Autodesk Inventor part; units mm, degrees
ref_plane "YZ Plane" through (0, 0, 0) normal (1, 0, 0) x (0, 1, 0)
ref_plane "XZ Plane" through (0, 0, 0) normal (0, 1, 0) x (-1, 0, 0)
ref_plane "XY Plane" through (0, 0, 0) normal (0, 0, 1) x (1, 0, 0)
sketch "スケッチ1" plane through (0, 0, 0) normal (0, 1, 0) x (-1, 0, 0)
  line L0 (0, 0) -> (0, -112.7681) construction
  line L1 (0, -112.7681) -> (0, 117.0869) construction
  line L2 (0, -1.5) -> (5, -1.5) construction
  line L3 (5, -1.5) -> (5, 1.5)
  line L4 (0, 1.5) -> (5, 1.5) construction
  line L5 (7.5, -1.5) -> (7.5, 1.5)
  line L6 (7.5, -1.5) -> (5, 1.5) construction
  line L7 (5, -1.5) -> (7.5, 1.5) construction
  line L8 (7.116, -1.5) -> (5.384, 1.5) construction
  line L9 (5.384, -1.5) -> (7.116, 1.5) construction
  line L10 (6.25, 0) -> (6.25, 1.5) construction
  line L11 (6.75, -0.866) -> (6.75, -1.5)
  line L12 (5.75, -0.866) -> (5.75, -1.5)
  line L13 (6.75, 0.866) -> (6.75, 1.5)
  line L14 (5.75, 0.866) -> (5.75, 1.5)
  line L15 (5, 1.5) -> (5.75, 1.5)
  line L16 (6.75, 1.5) -> (7.5, 1.5)
  arc A0 (6.75, 0.866) -> (5.75, 0.866) centre (6.25, 0) ccw
  arc A1 (5.75, 0.866) -> (5.75, -0.866) centre (6.25, 0) ccw
  arc A2 (5.75, -0.866) -> (6.8902, -0.7682) centre (6.25, 0) ccw
  arc A3 (6.8902, -0.7682) -> (6.75, 0.866) centre (6.25, 0) ccw
  line L17 (5, -1.5) -> (5.75, -1.5)
  line L18 (6.75, -1.5) -> (7.5, -1.5)
  point P0 (6.25, 0)
  dimension "d0" = 5
  dimension "d1" = 1.5
  dimension "d2" = 1.5
  dimension "d3" = 7.5
  dimension "d6" = 30
  dimension "d7" = 30
  dimension "d11" = 1
revolve "回転2" add sketch "スケッチ1" angle 360 about axis through (0, 0, 0) along (0, 0, -1)
properties part number "ベアリング10.15" material "ステンレス鋼"
The model under review builds one solid part; all positions refer to its coordinate system, in mm. Round coordinates to 2 decimals unless told otherwise and drop trailing zeros. Write each loop counter-clockwise with the first axis right and the second up, starting at its lowest first coordinate (ties: lowest second). Pieces come first, ordered by that corner, then holes.
(1) Insertion check: pin 1 (1.5 mm diameter, centred on y = 4, z = 0, fed in from -X). The pin has a flat end and moves straight along its axis. Give the tip position at first contact, or say it passes through.
(2) Mouldability with a two-part tool opening along Y and no side actions: class faces 1 (the cylindrical face through (0.75, 5.7, -1.19)), 2 (the cylindrical face through (7.493, -0.33, 0.021)), 3 (the flat face through (7, 1, 1.5)) as +Y half, -Y half, draft (parallel to the pull), parting line (faces both ways), or undercut.
(3) We need section A-A on x = 0. Give the boundary of the cut face in (y, z), and give its area (3 significant figures).
(4) We need section C-C on z = -0.2. Give the boundary of the cut face in (x, y), and give its area (3 significant figures).
(5) Wall thickness on L1, parallel to Y at x = 0, z = 1.1; L2, parallel to Y at x = 0, z = -0.55; L3, parallel to X at y = 4, z = 0.7: over which ranges is each line inside the solid? List them lowest first.
Findings below:
1. pin 1: stops at x = -6.76
2. face 1: undercut
2. face 2: parting line
2. face 3: draft
3. outline: (-7.5, -1.5) - (-6.75, -1.5) - (-6.75, -0.87) arc R1 ccw to (-5.75, -0.87) - (-5.75, -1.5) - (-5, -1.5) - (-5, 1.5) - (-5.75, 1.5) - (-5.75, 0.87) arc R1 ccw to (-6.75, 0.87) - (-6.75, 1.5) - (-7.5, 1.5) - close; (5, -1.5) - (5.75, -1.5) - (5.75, -0.87) arc R1 ccw to (6.75, -0.87) - (6.75, -1.5) - (7.5, -1.5) - (7.5, 1.5) - (6.75, 1.5) - (6.75, 0.87) arc R1 ccw to (5.75, 0.87) - (5.75, 1.5) - (5, 1.5) - close
3. area: 12.8 mm2
4. outline: circle Ø15 at (0, 0); hole circle Ø10 at (0, 0)
4. area: 98.2 mm2
5. L1: y = -7.5 to -6.75, -5.75 to -5, 5 to 5.75, 6.75 to 7.5
5. L2: y = -7.5 to -5, 5 to 7.5
5. L3: x = -6.34 to -3, 3 to 6.34
